```python
from build123d import *

# Parameters (mm, degrees)
BOSS_EXTRUDE1_DEPTH = 3.175


with BuildPart() as part:
    # Sketch1 → Boss-Extrude1 (new body)
    with BuildSketch(Plane.XY):
        with BuildLine():
            Line((98.429478474, -196.654958099), (98.429478474, -225.229958099))
            Line((98.429478474, -225.229958099), (-28.570521526, -225.229958099))
            Line((-28.570521526, -225.229958099), (-28.570521526, -123.629958099))
            Line((-28.570521526, -123.629958099), (25.404478474, -123.629958099))
            ThreePointArc((25.404478474, -123.629958099), (46.793005778, -175.266430795), (98.429478474, -196.654958099))
        make_face()
    extrude(amount=BOSS_EXTRUDE1_DEPTH)


solid = part.part
```
Input: part model. Units: mm. Frame: model coordinates. Give positions to 0.01 mm unless a question says otherwise; leave off trailing zeros. Loops run counter-clockwise (first coordinate to the right, second up) from the corner with the lowest first, then second, coordinate; pieces in that order, holes last. Notation, with made-up numbers: M 64,-11.75 L 105,-11.75 A23 cw 105,7.25 Z; hole C 72.25,0 d3. An arc over 180 degrees is marked long. Answer as CSV lines item,"result". Start each with the question number.
1. Pin query (flat end, axial travel): P1, Ø1.5, axis at y = -142, z = 0.5, coming from the +X side. Return the tip coordinate at first contact, or that it passes through.
2. Section A-A on z = 2.45. Return loops of the section in (x, y) (3 decimals), plus the area to 3 significant figures.
3. Section B-B on y = -160.5. Return loops of the section in (x, z) (3 decimals).
4. Line query: L1, parallel to Y at x = 46, z = 0.2; L2, parallel to X at y = -174.5, z = 0.6; L3, parallel to Y at x = 61, z = 0.2. Output: solid intervals per line, ascending.
5. Section C-C on x = 69. Return loops of the section in (y, z) (3 decimals).
Computed values:
1,P1,"stops at x = 27.95"
2,outline,"M -28.571,-225.23 L 98.429,-225.23 L 98.429,-196.655 A73.025 cw 25.404,-123.63 L -28.571,-123.63 Z"
2,area,"8,710 mm²"
3,outline,"M -28.571,0 L 35.396,0 L 35.396,3.175 L -28.571,3.175 Z"
4,L1,"y = -225.23 to -174.46"
4,L2,"x = -28.57 to 46.04"
4,L3,"y = -225.23 to -186.33"
5,outline,"M -225.23,0 L -190.462,0 L -190.462,3.175 L -225.23,3.175 Z"
